Design review of the part built by this model. Coordinates are the model's own, in mm. A direction names the side the tool comes from. Give positions to 0.01 mm unless a question says otherwise; leave off trailing zeros. Loops run counter-clockwise (first coordinate to the right, second up) from the corner with the lowest first, then second, coordinate; pieces in that order, holes last. Notation, with made-up numbers: (-3, -29) - (18, -29) arc R18 ccw to (18, 5) - close; hole circle Ø5 at (36.25, 74.25). An arc over 180 degrees is marked (long way). One line per item, written item: value. Start each with the question number.
```python
from build123d import *

# Parameters (mm, degrees)
BOSS_EXTRUDE1_DEPTH    = 2
BOSS_EXTRUDE2_DEPTH    = 4
CUT_EXTRUDE1_DEPTH     = 4
CIRPATTERN1_COUNT      = 2
LPATTERN4_COUNT        = 4
LPATTERN4_PITCH        = 29
LPATTERN4_COPY_1_DEPTH = 4
LPATTERN4_COPY_2_DEPTH = 4
LPATTERN4_COPY_3_DEPTH = 4
LPATTERN4_COPY_4_DEPTH = 4
LPATTERN4_COPY_5_DEPTH = 4
LPATTERN4_COPY_6_DEPTH = 4


with BuildPart() as part:
    # Sketch1 → Boss-Extrude1 (new body)
    with BuildSketch(Plane(origin=(0, 0, 0), x_dir=(1, 0, 0), z_dir=(0, 1, 0))):
        Polygon((-18, -58), (-18, -48), (-58, -48), (-58, 48), (-18, 48), (-18, 58), (22, 58), (22, 48), (58, 48), (58, -48), (22, -48), (22, -58), align=None)
    extrude(amount=BOSS_EXTRUDE1_DEPTH)

    # Sketch2 → Boss-Extrude2 (add)
    with BuildSketch(Plane(origin=(0, 0, -48), x_dir=(-1, 0, 0), z_dir=(0, 0, -1))):
        with BuildLine():
            Line((-58, 4.5), (-58, 2))
            Line((-58, 2), (-56.748331477, 2))
            ThreePointArc((-56.748331477, 2), (-56.5, 3.248331477), (-55.251668523, 3))
            Line((-55.251668523, 3), (-54.251668523, 3))
            Line((-54.251668523, 3), (-54.251668523, 4.5))
            Line((-54.251668523, 4.5), (-58, 4.5))
        make_face()
        with BuildLine():
            Line((-56.748331477, 2), (-58, 2))
            Line((-58, 2), (-58, 0))
            Line((-58, 0), (-54.251668523, 0))
            Line((-54.251668523, 0), (-54.251668523, 2))
            Line((-54.251668523, 2), (-55.251668523, 2))
            ThreePointArc((-55.251668523, 2), (-56, 1.6), (-56.748331477, 2))
        make_face()
    boss_extrude2 = extrude(amount=-BOSS_EXTRUDE2_DEPTH)

    # Sketch2_3 → Cut-Extrude1 (cut)
    with BuildSketch(Plane(origin=(0, 0, -48), x_dir=(-1, 0, 0), z_dir=(0, 0, -1))):
        with BuildLine():
            Line((-55.251668523, 2), (-56.748331477, 2))
            ThreePointArc((-56.748331477, 2), (-56, 1.6), (-55.251668523, 2))
        make_face()
    cut_extrude1 = extrude(amount=-CUT_EXTRUDE1_DEPTH, mode=Mode.SUBTRACT)

    # CirPattern1: Boss-Extrude2, Cut-Extrude1 ×2 about axis
    cirpattern1_axis = Axis((45.5, 0, 0), (0, 1, 0))
    add([boss_extrude2.rotate(cirpattern1_axis, i * 360 / CIRPATTERN1_COUNT) for i in range(1, CIRPATTERN1_COUNT)])
    add([cut_extrude1.rotate(cirpattern1_axis, i * 360 / CIRPATTERN1_COUNT) for i in range(1, CIRPATTERN1_COUNT)], mode=Mode.SUBTRACT)

    # LPattern4: Boss-Extrude2, Cut-Extrude1 ×4
    with Locations(*[(-i * LPATTERN4_PITCH, 0, 0) for i in range(1, LPATTERN4_COUNT)]):
        add(boss_extrude2)
        add(cut_extrude1, mode=Mode.SUBTRACT)

    # LPattern4 copy 1 sketch → LPattern4 copy 1 (add)
    with BuildSketch(Plane(origin=(62, 0, 48), x_dir=(1, 0, 0), z_dir=(0, 0, 1))):
        with BuildLine():
            Line((-58, 4.5), (-58, 2))
            Line((-58, 2), (-56.748331477, 2))
            ThreePointArc((-56.748331477, 2), (-56.5, 3.248331477), (-55.251668523, 3))
            Line((-55.251668523, 3), (-54.251668523, 3))
            Line((-54.251668523, 3), (-54.251668523, 4.5))
            Line((-54.251668523, 4.5), (-58, 4.5))
        make_face()
        with BuildLine():
            Line((-56.748331477, 2), (-58, 2))
            Line((-58, 2), (-58, 0))
            Line((-58, 0), (-54.251668523, 0))
            Line((-54.251668523, 0), (-54.251668523, 2))
            Line((-54.251668523, 2), (-55.251668523, 2))
            ThreePointArc((-55.251668523, 2), (-56, 1.6), (-56.748331477, 2))
        make_face()
    extrude(amount=-LPATTERN4_COPY_1_DEPTH)

    # LPattern4 copy 2 sketch → LPattern4 copy 2 (add)
    with BuildSketch(Plane(origin=(33, 0, 48), x_dir=(1, 0, 0), z_dir=(0, 0, 1))):
        with BuildLine():
            Line((-58, 4.5), (-58, 2))
            Line((-58, 2), (-56.748331477, 2))
            ThreePointArc((-56.748331477, 2), (-56.5, 3.248331477), (-55.251668523, 3))
            Line((-55.251668523, 3), (-54.251668523, 3))
            Line((-54.251668523, 3), (-54.251668523, 4.5))
            Line((-54.251668523, 4.5), (-58, 4.5))
        make_face()
        with BuildLine():
            Line((-56.748331477, 2), (-58, 2))
            Line((-58, 2), (-58, 0))
            Line((-58, 0), (-54.251668523, 0))
            Line((-54.251668523, 0), (-54.251668523, 2))
            Line((-54.251668523, 2), (-55.251668523, 2))
            ThreePointArc((-55.251668523, 2), (-56, 1.6), (-56.748331477, 2))
        make_face()
    extrude(amount=-LPATTERN4_COPY_2_DEPTH)

    # LPattern4 copy 3 sketch → LPattern4 copy 3 (add)
    with BuildSketch(Plane(origin=(4, 0, 48), x_dir=(1, 0, 0), z_dir=(0, 0, 1))):
        with BuildLine():
            Line((-58, 4.5), (-58, 2))
            Line((-58, 2), (-56.748331477, 2))
            ThreePointArc((-56.748331477, 2), (-56.5, 3.248331477), (-55.251668523, 3))
            Line((-55.251668523, 3), (-54.251668523, 3))
            Line((-54.251668523, 3), (-54.251668523, 4.5))
            Line((-54.251668523, 4.5), (-58, 4.5))
        make_face()
        with BuildLine():
            Line((-56.748331477, 2), (-58, 2))
            Line((-58, 2), (-58, 0))
            Line((-58, 0), (-54.251668523, 0))
            Line((-54.251668523, 0), (-54.251668523, 2))
            Line((-54.251668523, 2), (-55.251668523, 2))
            ThreePointArc((-55.251668523, 2), (-56, 1.6), (-56.748331477, 2))
        make_face()
    extrude(amount=-LPATTERN4_COPY_3_DEPTH)

    # LPattern4 copy 4 sketch → LPattern4 copy 4 (cut)
    with BuildSketch(Plane(origin=(62, 0, 48), x_dir=(1, 0, 0), z_dir=(0, 0, 1))):
        with BuildLine():
            Line((-55.251668523, 2), (-56.748331477, 2))
            ThreePointArc((-56.748331477, 2), (-56, 1.6), (-55.251668523, 2))
        make_face()
    extrude(amount=-LPATTERN4_COPY_4_DEPTH, mode=Mode.SUBTRACT)

    # LPattern4 copy 5 sketch → LPattern4 copy 5 (cut)
    with BuildSketch(Plane(origin=(33, 0, 48), x_dir=(1, 0, 0), z_dir=(0, 0, 1))):
        with BuildLine():
            Line((-55.251668523, 2), (-56.748331477, 2))
            ThreePointArc((-56.748331477, 2), (-56, 1.6), (-55.251668523, 2))
        make_face()
    extrude(amount=-LPATTERN4_COPY_5_DEPTH, mode=Mode.SUBTRACT)

    # LPattern4 copy 6 sketch → LPattern4 copy 6 (cut)
    with BuildSketch(Plane(origin=(4, 0, 48), x_dir=(1, 0, 0), z_dir=(0, 0, 1))):
        with BuildLine():
            Line((-55.251668523, 2), (-56.748331477, 2))
            ThreePointArc((-56.748331477, 2), (-56, 1.6), (-55.251668523, 2))
        make_face()
    extrude(amount=-LPATTERN4_COPY_6_DEPTH, mode=Mode.SUBTRACT)


solid = part.part
```
(1) To check wall thickness, follow L1, parallel to Y at x = 45, z = 37.5; L2, parallel to X at y = 1.7, z = 53.5; L3, parallel to Z at x = 51, y = 0.9. State the ranges of each line that lie inside material, in increasing order. Write a range as from..to.
(2) Machinability: for faces 1 (the flat face through (5, 4, 44)), 2 (the flat face through (28, 4, -44)), 3 (the flat face through (40, 1, -48)), 4 (the flat face through (0, 3, -46)), 5 (the flat face through (40, 1, 48)), which of the approach directions +Z, -Z, +X, -X, +Y, -Y give a long, thin tool a straight path to every point of the face, cutting with its end or side? Answer none if there is none.
(3) Draft analysis for pull direction X (two halves, no side actions). For faces 6 (the flat face through (33, 3, 46)), 7 (the flat face through (-30, 4, -44)), 8 (the flat face through (58, 1, -1)), state which applies: pulls with the +X half, pulls with the -X half, needs draft (parallel to the pull), parting line crosses it, or undercut.
(4) Take a section at B-B on z = -38.5. State the section outline as (x, y) points, and give its area (3 significant figures).
(5) Take a section at A-A on y = 0.7. State the section outline as (x, z) points, and give its area (3 significant figures).
(6) For pin 1 Ø1.2 at (x, y) = (27, 4) entering from +Z; pin 2 Ø2 at (y, z) = (1, -51) entering from +X; pin 3 Ø0.8 at (x, y) = (-23.5, 3.5) entering from -Z; pin 4 Ø6 at (x, z) = (36.5, -46.5) entering from -Y, all flat-tipped, find the tip position at first contact; note any pin that passes through.
Here are the results:
1. L1: 0..2
1. L2: -18..22
1. L3: -48..48
2. face 1: -Z, +X, -X, +Y
2. face 2: +Z, +X, -X, +Y
2. face 3: -Z, +X, +Y, -Y
2. face 4: +Z, -Z, +Y
2. face 5: +Z, +X, +Y, -Y
3. face 6: undercut
3. face 7: needs draft
3. face 8: pulls with the +X half
4. outline: (-58, 0) - (58, 0) - (58, 2) - (-58, 2) - close
4. area: 232 mm²
5. outline: (-58, -48) - (-18, -48) - (-18, -58) - (22, -58) - (22, -48) - (58, -48) - (58, 48) - (22, 48) - (22, 58) - (-18, 58) - (-18, 48) - (-58, 48) - close
5. area: 11,900 mm²
6. pin 1: z = -44
6. pin 2: x = 22
6. pin 3: z = 44
6. pin 4: y = 0
